```python
from build123d import *

# Parameters (mm, degrees)
F1_DEPTH = 10
F2_W     = 14
F2_H     = 2
F3_DEPTH = 10
F4_R     = 1.5
F5_DEPTH = 25
F6_R     = 4.99999


# Not quite as in the source:
# - a fillet or chamfer is up to 0.001 mm smaller than in the source, because OpenCascade refuses the exact size


with BuildPart() as f1:
    # F0 (on Top) → F1 (new body)
    with BuildSketch(Plane.XY):
        Polygon((4, 0), (0, 0), (-4, 0), (-6, 0), (-6, -2), (6, -2), (6, 0), align=None)
        Polygon((-6, 0), (-4, 0), (-4, 12), (-2.2325584196, 15.5), (2.2325584196, 15.5), (4, 12), (4, 0), (6, 0), (6, 17.5), (-6, 17.5), align=None)
    extrude(amount=F1_DEPTH)

    # F2 (on face) → F3 (join)
    with BuildSketch(Plane.XY.offset(10)):
        with Locations((-13, -1)):
            Rectangle(F2_W, F2_H)
        with Locations((13, -1)):
            Rectangle(F2_W, F2_H)
    extrude(amount=-F3_DEPTH)

    # F4 (on face) → F5 (cut)
    with BuildSketch(Plane(origin=(0, 0, 0), x_dir=(-1, 0, 0), z_dir=(0, 1, 0))):
        with Locations((16.25, 5)):
            Circle(F4_R)
        with Locations((-16.25, 5)):
            Circle(F4_R)
    extrude(amount=-F5_DEPTH, mode=Mode.SUBTRACT)

    # F6 (radius 5 in the source; OpenCascade refuses exactly that, so slightly less here)
    f6_edges = [f1.edges().sort_by_distance(p)[0] for p in [
        (-6, 17.5, 5),
        (6, 17.5, 5),
        (-6, 0, 5),
        (6, 0, 5),
        (-20, -1, 10),
        (-20, -1, 0),
        (20, -1, 10),
        (20, -1, 0),
    ]]
    fillet(f6_edges, radius=F6_R)


solid = f1.part
```
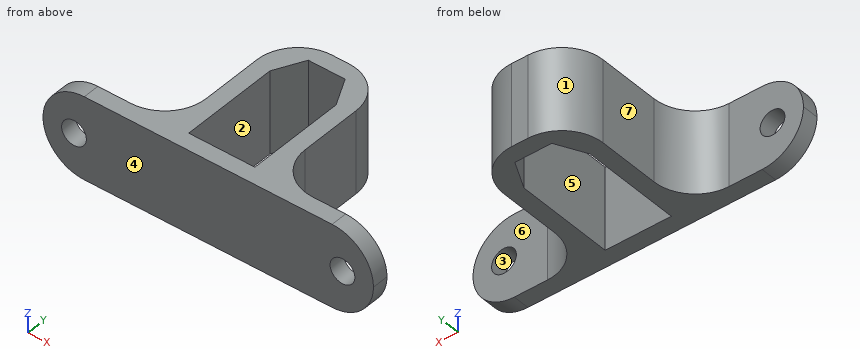
For this review, take the finished solid that the model builds, in its own axes (mm). Face numbers are marked on the shaded views. A direction names the side the tool comes from. Coordinates: 2 decimals unless noted, no trailing zeros. Order: outer loops, then holes, each group sorted by start corner. A loop starts at its lowest first (then second) coordinate and runs counter-clockwise, first axis right, second up. Notation, with made-up numbers: (43, 62) -> (49, 62) arc R11 ccw to (49, 78) -> close; hole circle Ø6 at (-37.5, 70). An arc over 180 degrees is marked (long way). Use CSV: the item, a comma, the result in double quotes. Start each with the question number.
Item 1: Wall thickness on probe 1 along Y at (x, z) = (-1, 9.75); probe 2 along X at (y, z) = (11.5, 1); probe 3 along Y at (x, z) = (-12, 7.5): over which ranges is each line inside the solid? List them lowest first.
Item 2: We need section C-C, the plane z = 4. Give the boundary of the cut face in (x, y), then the cut area to 3 significant figures.
Item 3: We need section D-D, the plane z = 9.25. Give the boundary of the cut face in (x, y), then the cut area to 3 significant figures.
Item 4: Draft analysis for pull direction Y (two halves, no side actions). For the marked faces 1, 2, 3 and 4, state which applies: pulls with the +Y half, pulls with the -Y half, needs draft (parallel to the pull), parting line crosses it, or undercut.
Item 5: We need section A-A, the plane y = 11. Give the boundary of the cut face in (x, z).
Item 6: Insertion check: pin 1 (4 mm diameter, centred on x = 9.5, y = 4, fed in from -Z); pin 2 (5 mm diameter, centred on y = 8, z = 3.5, fed in from -X); pin 3 (2 mm diameter, centred on y = 4, z = 7.5, fed in from -X); pin 4 (2.5 mm diameter, centred on y = 9, z = 6.5, fed in from +X). Each pin has a flat end and moves straight along its axis. Give the tip position at first contact, or say it passes through.
Item 7: We need section B-B, the plane x = -1.5. Give the boundary of the cut face in (y, z).
Item 8: For the marked faces 5, 6 and 7, list the 3-axis set-ups (+Z, -Z, +X, -X, +Y, -Y) from which the entire face can be reached by the end or side of a thin tool; tool diameter is ignored.
Derived:
1,probe 1,"y = -2 to 0, 15.5 to 17.5"
1,probe 2,"x = -6 to -4, 4 to 6"
1,probe 3,"y = -2 to 0"
2,outline,"(-19.9, -2) -> (-17.37, -2) -> (-17.37, 0) -> (-19.9, 0) -> close; (-15.13, -2) -> (15.13, -2) -> (15.13, 0) -> (11, 0) arc R5 cw to (6, 5) -> (6, 12.5) arc R5 ccw to (1, 17.5) -> (-1, 17.5) arc R5 ccw to (-6, 12.5) -> (-6, 5) arc R5 cw to (-11, 0) -> (-15.13, 0) -> close; (17.37, -2) -> (19.9, -2) -> (19.9, 0) -> (17.37, 0) -> close; hole (-4, 0) -> (4, 0) -> (4, 12) -> (2.23, 15.5) -> (-2.23, 15.5) -> (-4, 12) -> close"
2,area,"163 mm^2"
3,outline,"(-17.63, -2) -> (17.63, -2) -> (17.63, 0) -> (11, 0) arc R5 cw to (6, 5) -> (6, 12.5) arc R5 ccw to (1, 17.5) -> (-1, 17.5) arc R5 ccw to (-6, 12.5) -> (-6, 5) arc R5 cw to (-11, 0) -> (-17.63, 0) -> close; hole (-4, 0) -> (4, 0) -> (4, 12) -> (2.23, 15.5) -> (-2.23, 15.5) -> (-4, 12) -> close"
3,area,"163 mm^2"
4,face 1,"pulls with the +Y half"
4,face 2,"undercut"
4,face 3,"needs draft"
4,face 4,"pulls with the -Y half"
5,outline,"(-6, 0) -> (-4, 0) -> (-4, 10) -> (-6, 10) -> close; (4, 0) -> (6, 0) -> (6, 10) -> (4, 10) -> close"
6,pin 1,"passes through"
6,pin 2,"stops at x = -6"
6,pin 3,"stops at x = -6.42"
6,pin 4,"stops at x = 6"
7,outline,"(-2, 0) -> (0, 0) -> (0, 10) -> (-2, 10) -> close; (15.5, 0) -> (17.47, 0) -> (17.47, 10) -> (15.5, 10) -> close"
8,face 5,"+Z, -Z"
8,face 6,"+Z, -Z, +X, +Y"
8,face 7,"+Z, -Z, -X, +Y"
